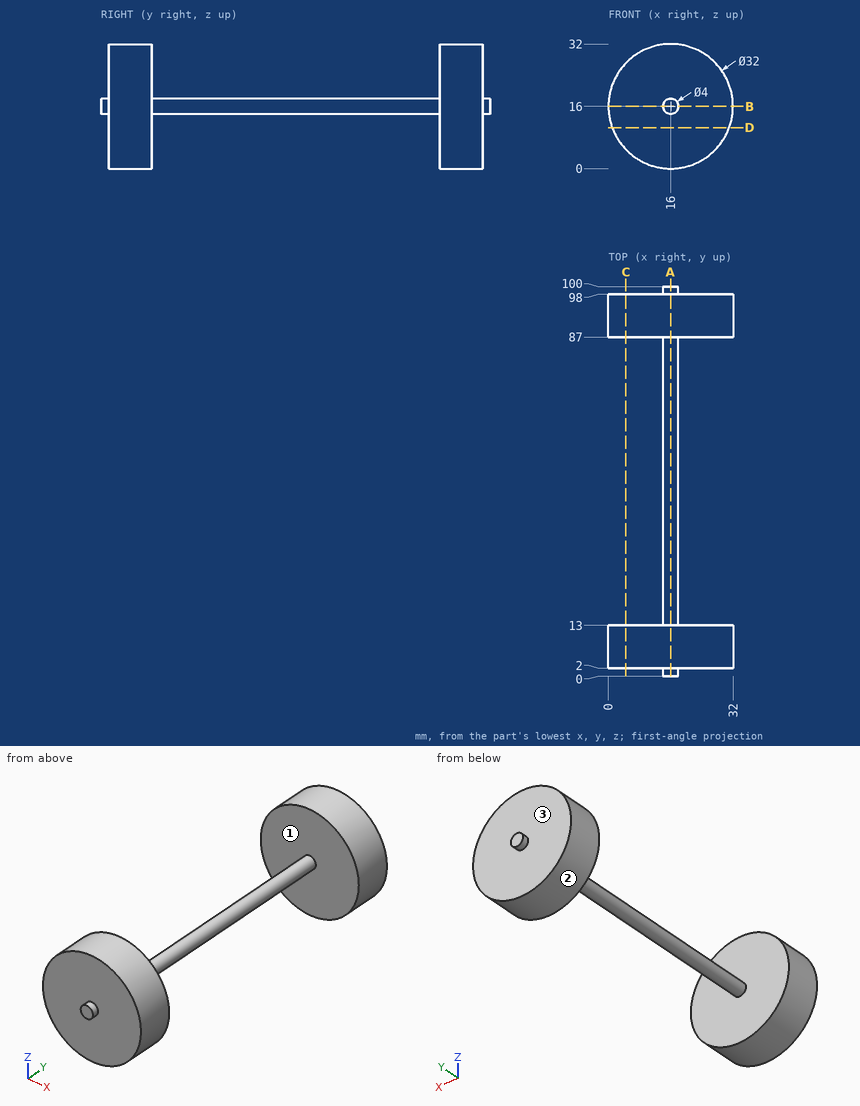
Geometry: see drawing. Coordinates: mm, zero at the bounding-box minimum. Round coordinates to 2 decimals unless told otherwise and drop trailing zeros. Write each loop counter-clockwise with the first axis right and the second up, starting at its lowest first coordinate (ties: lowest second). Pieces come first, ordered by that corner, then holes.
Item 1: Section query A-A (x = 16). Return loops of the section in (y, z).
Item 2: Section query B-B (z = 16). Return loops of the section in (x, y), plus the area to 3 significant figures.
Item 3: Section query D-D (z = 10.5). Return loops of the section in (x, y).
Item 4: Section query C-C (x = 4.5). Return loops of the section in (y, z), plus the area to 3 significant figures.
Item 5: Mould query, pull axis Y, two halves, no side actions, for the marked faces 1, 2 and 3. Classes: +Y half, -Y half, draft (parallel to the pull), parting line (faces both ways), or undercut.
Item 6: Pin query (flat end, axial travel): P1, Ø12, axis at x = 19.5, z = 26.5, coming from the +Y side; P2, Ø5, axis at x = 8, z = 25, coming from the -Y side; P3, Ø12, axis at y = 77.5, z = 13, coming from the +X side. Return the tip coordinate at first contact, or that it passes through.
Item 7: Material intervals for L1, parallel to Y at x = 5.5, z = 24.5; L2, parallel to X at y = 54.5, z = 15; L3, parallel to Z at x = 26, y = 87.5, sorted ascending.
Completed:
1. outline: (0, 14) - (2, 14) - (2, 0) - (13, 0) - (13, 14) - (87, 14) - (87, 0) - (98, 0) - (98, 14) - (100, 14) - (100, 18) - (98, 18) - (98, 32) - (87, 32) - (87, 18) - (13, 18) - (13, 32) - (2, 32) - (2, 18) - (0, 18) - close
2. outline: (0, 2) - (14, 2) - (14, 0) - (18, 0) - (18, 2) - (32, 2) - (32, 13) - (18, 13) - (18, 87) - (32, 87) - (32, 98) - (18, 98) - (18, 100) - (14, 100) - (14, 98) - (0, 98) - (0, 87) - (14, 87) - (14, 13) - (0, 13) - close
2. area: 1,020 mm2
3. outline: (0.98, 2) - (31.02, 2) - (31.02, 13) - (0.98, 13) - close; (0.98, 87) - (31.02, 87) - (31.02, 98) - (0.98, 98) - close
4. outline: (2, 4.88) - (13, 4.88) - (13, 27.12) - (2, 27.12) - close; (87, 4.88) - (98, 4.88) - (98, 27.12) - (87, 27.12) - close
4. area: 489 mm2
5. face 1: undercut
5. face 2: draft
5. face 3: +Y half
6. P1: stops at y = 98
6. P2: stops at y = 2
6. P3: stops at x = 18
7. L1: y = 2 to 13, 87 to 98
7. L2: x = 14.27 to 17.73
7. L3: z = 3.51 to 28.49
